```python
from build123d import *

# Parameters (mm, degrees)
SKETCH_1_W           = 270
SKETCH_1_H           = 370
SKETCH_1_W_2         = 250
SKETCH_1_H_2         = 350
EXTRUDE_2_DEPTH      = 45
SKETCH_4_W           = 250
SKETCH_4_H           = 350
SKETCH_4_W_2         = 222
SKETCH_4_H_2         = 322
EXTRUDE_3_DEPTH      = 5
SKETCH_9_W           = 246
SKETCH_9_H           = 346
SKETCH_9_W_2         = 226
SKETCH_9_H_2         = 326
CUT_EXTRUDE_3_DEPTH  = 2.5
SKETCH_12_R          = 1.6
CUT_EXTRUDE_5_DEPTH  = 109.5
FILLET_1_R           = 5
SKETCH_13_W          = 250
SKETCH_13_H          = 350
SKETCH_13_W_2        = 222
SKETCH_13_H_2        = 322
EXTRUDE_4_DEPTH      = 33.5
CUT_EXTRUDE_START    = -126.5
SKETCH_14_R          = 1.6
CUT_EXTRUDE_8_DEPTH  = 126.5
SKETCH_15_W          = 209.875644348
SKETCH_15_H          = 2
CUT_EXTRUDE_9_DEPTH  = 2.5
CUT_EXTRUDE_10_DEPTH = 60.5
SKETCH_18_R          = 1.6
CUT_EXTRUDE_11_DEPTH = 60.5
SKETCH_21_R          = 3
CUT_EXTRUDE_14_DEPTH = 40


with BuildPart() as part:
    # Sketch 1 → Extrude 2 (new body)
    with BuildSketch(Plane(origin=(0, 0, 0), x_dir=(1, 0, 0), z_dir=(0, 1, 0))):
        with Locations((125, 175)):
            Rectangle(SKETCH_1_W, SKETCH_1_H)
        with Locations((125, 175)):
            Rectangle(SKETCH_1_W_2, SKETCH_1_H_2, mode=Mode.SUBTRACT)
    extrude(amount=EXTRUDE_2_DEPTH)

    # Sketch 4 → Extrude 3 (add)
    with BuildSketch(Plane(origin=(0, 38.5, 0), x_dir=(1, 0, 0), z_dir=(0, 1, 0))):
        with Locations((125, 175)):
            Rectangle(SKETCH_4_W, SKETCH_4_H)
        with Locations((125, 175)):
            Rectangle(SKETCH_4_W_2, SKETCH_4_H_2, mode=Mode.SUBTRACT)
    extrude(amount=-EXTRUDE_3_DEPTH)

    # Sketch 9 → Cut-Extrude 3 (cut)
    with BuildSketch(Plane(origin=(0, 38.5, 0), x_dir=(1, 0, 0), z_dir=(0, 1, 0))):
        with Locations((125, 175)):
            Rectangle(SKETCH_9_W, SKETCH_9_H)
        with Locations((125, 175)):
            Rectangle(SKETCH_9_W_2, SKETCH_9_H_2, mode=Mode.SUBTRACT)
    extrude(amount=-CUT_EXTRUDE_3_DEPTH, mode=Mode.SUBTRACT)

    # Sketch 12 → Cut-Extrude 5 (cut)
    with BuildSketch(Plane(origin=(0, 45, 0), x_dir=(1, 0, 0), z_dir=(0, 1, 0))):
        with Locations(Location((-5, -5, 0), (0, 0, 270))):
            Circle(SKETCH_12_R)
        with BuildLine():
            ThreePointArc((-6.13137085, 356.13137085), (-6.13137085, 353.86862915), (-3.86862915, 353.86862915))
            Line((-3.86862915, 353.86862915), (-6.13137085, 356.13137085))
        make_face()
        with BuildLine():
            Line((-6.13137085, 356.13137085), (-3.86862915, 353.86862915))
            ThreePointArc((-3.86862915, 353.86862915), (-3.521792748, 354.387706508), (-3.4, 355))
            ThreePointArc((-3.4, 355), (-4.387706508, 356.478207252), (-6.13137085, 356.13137085))
        make_face()
        with Locations(Location((255, 355, 0), (0, 0, 270))):
            Circle(SKETCH_12_R)
        with Locations(Location((255, -5, 0), (0, 0, 270))):
            Circle(SKETCH_12_R)
    extrude(amount=-CUT_EXTRUDE_5_DEPTH, mode=Mode.SUBTRACT)

    # Fillet 1
    fillet_1_edges = [part.edges().sort_by_distance(p)[0] for p in [
        (-10, 22.5, 10),
        (-10, 22.5, -360),
        (260, 22.5, -360),
        (260, 22.5, 10),
    ]]
    fillet(fillet_1_edges, radius=FILLET_1_R)

    # Sketch 13 → Extrude 4 (add)
    with BuildSketch(Plane.XZ.offset(-33.5)):
        with Locations((125, -175)):
            Rectangle(SKETCH_13_W, SKETCH_13_H)
        with Locations((125, -175)):
            Rectangle(SKETCH_13_W_2, SKETCH_13_H_2, mode=Mode.SUBTRACT)
    extrude(amount=EXTRUDE_4_DEPTH)

    # Sketch 14 → Cut-Extrude 8 (cut)
    # profile 1 of 7: a face of its own
    with BuildSketch(Plane.XZ.offset(CUT_EXTRUDE_START)):
        with BuildLine():
            Line((14, -336), (14, -14))
            Line((14, -14), (14, -6))
            Line((14, -6), (14, 2))
            Line((14, 2), (14, 10))
            Line((14, 10), (-5, 10))
            ThreePointArc((-5, 10), (-8.535533906, 8.535533906), (-10, 5))
            Line((-10, 5), (-10, -355))
            ThreePointArc((-10, -355), (-8.535533906, -358.535533906), (-5, -360))
            Line((-5, -360), (255, -360))
            ThreePointArc((255, -360), (258.535533906, -358.535533906), (260, -355))
            Line((260, -355), (260, 5))
            ThreePointArc((260, 5), (258.535533906, 8.535533906), (255, 10))
            Line((255, 10), (236, 10))
            Line((236, 10), (236, 2))
            Line((236, 2), (236, -6))
            Line((236, -6), (236, -14))
            Line((236, -14), (236, -336))
            Line((236, -336), (14, -336))
        make_face()
        with Locations((-5, -355)):
            Circle(SKETCH_14_R, mode=Mode.SUBTRACT)
        with Locations((255, -355)):
            Circle(SKETCH_14_R, mode=Mode.SUBTRACT)
        with Locations((-5, 5)):
            Circle(SKETCH_14_R, mode=Mode.SUBTRACT)
        with Locations((255, 5)):
            Circle(SKETCH_14_R, mode=Mode.SUBTRACT)
    # profile 2 of 7: a face of its own
    with BuildSketch(Plane.XZ.offset(CUT_EXTRUDE_START)):
        Polygon((14, 2), (14, -6), (20.062177826, -9.5), (20.062177826, 5.5), align=None)
    # profile 3 of 7: a face of its own
    with BuildSketch(Plane.XZ.offset(CUT_EXTRUDE_START)):
        with Locations((-5, 5)):
            Circle(SKETCH_14_R)
    # profile 4 of 7: a face of its own
    with BuildSketch(Plane.XZ.offset(CUT_EXTRUDE_START)):
        Polygon((229.937822174, -9.5), (236, -6), (236, 2), (229.937822174, 5.5), align=None)
    # profile 5 of 7: a face of its own
    with BuildSketch(Plane.XZ.offset(CUT_EXTRUDE_START)):
        with Locations((255, 5)):
            Circle(SKETCH_14_R)
    # profile 6 of 7: a face of its own
    with BuildSketch(Plane.XZ.offset(CUT_EXTRUDE_START)):
        with Locations((255, -355)):
            Circle(SKETCH_14_R)
    # profile 7 of 7: a face of its own
    with BuildSketch(Plane.XZ.offset(CUT_EXTRUDE_START)):
        with Locations((-5, -355)):
            Circle(SKETCH_14_R)
    extrude(amount=CUT_EXTRUDE_8_DEPTH, mode=Mode.SUBTRACT)

    # Sketch 15 → Cut-Extrude 9 (cut)
    with BuildSketch(Plane(origin=(0, 38.5, 0), x_dir=(1, 0, 0), z_dir=(0, 1, 0))):
        with Locations((125, 1)):
            Rectangle(SKETCH_15_W, SKETCH_15_H)
    extrude(amount=-CUT_EXTRUDE_9_DEPTH, mode=Mode.SUBTRACT)

    # Sketch 16 → Cut-Extrude 10 (cut)
    with BuildSketch(Plane(origin=(0, 45, 0), x_dir=(1, 0, 0), z_dir=(0, 1, 0))):
        Polygon((236, -10), (236, -8), (234, -8), (229.607695155, -8), (14, -8), (14, -10), align=None)
    extrude(amount=-CUT_EXTRUDE_10_DEPTH, mode=Mode.SUBTRACT)

    # Sketch 18 → Cut-Extrude 11 (cut)
    with BuildSketch(Plane(origin=(0, 45, 0), x_dir=(1, 0, 0), z_dir=(0, 1, 0))):
        with Locations(Location((166, -4, 0), (0, 0, 270))):
            Circle(SKETCH_18_R)
        with Locations(Location((84, -4, 0), (0, 0, 270))):
            Circle(SKETCH_18_R)
    extrude(amount=-CUT_EXTRUDE_11_DEPTH, mode=Mode.SUBTRACT)

    # Sketch 21 → Cut-Extrude 14 (cut)
    with BuildSketch(Plane(origin=(0, 0, -14), x_dir=(-1, 0, 0), z_dir=(0, 0, -1))):
        with Locations((-206, 19.25)):
            Circle(SKETCH_21_R)
    extrude(amount=-CUT_EXTRUDE_14_DEPTH, mode=Mode.SUBTRACT)


solid = part.part
```
Check sheet for the modelled part. Datum: model origin and axes. Units: mm. A direction names the side the tool comes from. Coordinates: 2 decimals unless noted, no trailing zeros. Write each loop counter-clockwise with the first axis right and the second up, starting at its lowest first coordinate (ties: lowest second). Pieces come first, ordered by that corner, then holes. Notation, with made-up numbers: M 76,-19 L 103,-19 A18 cw 103,1 Z; hole C -19.75,65 d11. An arc over 180 degrees is marked long. Use one line per item in the form item = value.
Item 1: Gauge pin test, flat ends, axial feed: pin 1 Ø6 at (x, z) = (128, -5) entering from +Y; pin 2 Ø1.6 at (x, z) = (101, -13) entering from +Y. Record the tip position at first contact, or that the pin passes through.
Answer below:
pin_1 = 36
pin_2 = 38.5
Item 2: Sectioned sample at D-D, the plane x = 54.5. Record the cut outline in (y, z).
Answer below:
outline = M 0,-14 L 38.5,-14 L 38.5,-12 L 36,-12 L 36,0 L 45,0 L 45,8 L 0,8 Z
Item 3: Sectioned sample at A-A, the plane y = 19.25. Record the cut outline in (x, z).
Answer below:
outline = M 14,-14 L 203,-14 L 203,8 L 14,8 L 14,2 L 20.06,5.5 L 20.06,-9.5 L 14,-6 Z; M 209,-14 L 236,-14 L 236,-6 L 229.94,-9.5 L 229.94,5.5 L 236,2 L 236,8 L 209,8 Z; hole C 84,4 d3.2; hole C 166,4 d3.2
Item 4: Release check for a two-part mould opening along X. For faces 1 (the face through (236, 20, -10)), 2 (the face through (208.381, 17.425, -3.154)), 3 (the face through (14, 20, -10)), 4 (the face through (123, 45, 4)) record: pulls with the +X half, pulls with the -X half, needs draft (parallel to the pull), parting line crosses it, or undercut.
Answer below:
face_1 = pulls with the +X half
face_2 = undercut
face_3 = pulls with the -X half
face_4 = needs draft
Item 5: Material ranges on L1, parallel to Y at x = 206, z = -9.5; L2, parallel to Y at x = 206, z = 1.5; L3, parallel to Z at x = 84, y = 34, recorded low to high. Write a range as from..to.
Answer below:
L1 = 0..16.25, 22.25..36
L2 = 0..16.25, 22.25..45
L3 = -14..2.4, 5.6..8
Item 6: Set-up check for faces 5 (the face through (236, 23, 5)), 6 (the face through (123, 36, -6)): record each of +Z, -Z, +X, -X, +Y, -Y from which the full face is reachable in a straight line by a thin tool's end or side.
Answer below:
face_5 = +Z, -Z, +X, +Y, -Y
face_6 = +X, -X, +Y
Item 7: Sectioned sample at B-B, the plane x = 206. Record the cut outline in (y, z).
Answer below:
outline = M 0,-14 L 16.25,-14 L 16.25,8 L 0,8 Z; M 22.25,-14 L 38.5,-14 L 38.5,-12 L 36,-12 L 36,0 L 45,0 L 45,8 L 22.25,8 Z
Item 8: Sectioned sample at C-C, the plane y = 6.5. Record the cut outline in (x, z).
Answer below:
outline = M 14,-14 L 236,-14 L 236,-6 L 229.94,-9.5 L 229.94,5.5 L 236,2 L 236,8 L 14,8 L 14,2 L 20.06,5.5 L 20.06,-9.5 L 14,-6 Z; hole C 84,4 d3.2; hole C 166,4 d3.2
